Build history of the part. All positions in model axes, mm. A direction names the side the tool comes from. Coordinates: 2 decimals unless noted, no trailing zeros. Loops run counter-clockwise (first coordinate to the right, second up) from the corner with the lowest first, then second, coordinate; pieces in that order, holes last. Notation, with made-up numbers: (74.5, -32.75) -> (133.5, -32.75) arc R24 ccw to (133.5, -5.75) -> close; hole circle Ø3 at (29, 46.25). An arc over 180 degrees is marked (long way). One line per item, written item: value. Start each with the question number.
```python
from build123d import *

# Parameters (mm, degrees)
ESQUISSE6_R        = 25
ESQUISSE6_R_2      = 24
ESQUISSE8_R        = 26.000000000000004
ESQUISSE8_R_2      = 24.000000000000004
EXTRU_MINCE1_DEPTH = 1
EXTRU_MINCE2_START = 30
ESQUISSE9_R        = 26
ESQUISSE9_R_2      = 25
EXTRU_MINCE2_DEPTH = 30
CONG_1_R           = 1
CONG_2_R           = 1


with BuildPart() as part:
    # Balayage-Mince2: sweep along a path in Esquisse7
    with BuildLine(Plane(origin=(0, 0, 0), x_dir=(0, 0, -1), z_dir=(1, 0, 0))) as balayage_mince2_path:
        Line((0, 0), (-64.71019057874605, -6.94e-15))
        ThreePointArc((-64.71019057874605, -6.94e-15), (-69.91963590875396, 0.45576740963375073), (-74.97079487851613, 1.8092213764227365))
        Line((-74.97079487851613, 1.8092213764227365), (-106.64801221065042, 13.338785589701102))
    # Esquisse6 → Balayage-Mince2 (sweep)
    with BuildSketch(Plane.XY):
        Circle(ESQUISSE6_R)
        Circle(ESQUISSE6_R_2, mode=Mode.SUBTRACT)
    sweep(path=balayage_mince2_path.line)



with BuildPart() as body_2:
    # Esquisse8 → Extru.-Mince1 (new body)
    with BuildSketch(Plane(origin=(0, 35.836351928730004, 98.45956771981464), x_dir=(1, 0, 0), z_dir=(0, 0.34202014332566966, 0.9396926207859081))):
        with Locations((0, -23.94141003279684)):
            Circle(ESQUISSE8_R)
        with Locations((0, -23.94141003279684)):
            Circle(ESQUISSE8_R_2, mode=Mode.SUBTRACT)
    extrude(amount=EXTRU_MINCE1_DEPTH)


with BuildPart() as part_1:
    add(part.part)

    add(body_2.part)  # Extru.-Mince2 merges body 2
    # Esquisse9 → Extru.-Mince2 (add)
    with BuildSketch(Plane(origin=(0, 36.17837207205572, 99.39926034060053), x_dir=(1, 0, 0), z_dir=(0, 0.3420201433256696, 0.9396926207859081)).offset(EXTRU_MINCE2_START)):
        with Locations((0, -23.941410032796895)):
            Circle(ESQUISSE9_R)
        with Locations((0, -23.941410032796895)):
            Circle(ESQUISSE9_R_2, mode=Mode.SUBTRACT)
    extrude(amount=-EXTRU_MINCE2_DEPTH)

    # Congé1
    cong_1_edges = [part_1.edges().sort_by_distance(p)[0] for p in [
        (-25, 13.338785589701132, 106.6480122106504),
    ]]
    fillet(cong_1_edges, radius=CONG_1_R - 0.0001)  # a hair under: the kernel refuses the full size

    # Congé2
    cong_2_edges = [part_1.edges().sort_by_distance(p)[0] for p in [
        (-26.000000000000004, 13.33878558970111, 106.64801221065045),
    ]]
    fillet(cong_2_edges, radius=CONG_2_R)


solid = part_1.part
```
Item 1: Band-saw the part on A-A, the plane z = 50. List the corners of the cut face in (x, y), and give its area (3 significant figures).
Item 2: Tool access for faces 4 (the face through (-23.977, 1.055, 32.808)), 5 (the face through (-22.34, 22.49, 104.38)), 6 (the face through (-13.603, 43.963, 128.491)): list every direction of +Z, -Z, +X, -X, +Y, -Y with a clear straight run to the whole face (end or side of a thin tool).
Item 3: Probe probe 1 along Y at (x, z) = (0, 35); probe 2 along Y at (x, z) = (-4.5, 97); probe 3 along X at (y, z) = (3, 72). List the from-to ranges inside material, lowest first.
Item 4: Two-plate mould, pull along X, no slides. Class faces 1 (the face through (23.846, 25.939, 119.312)), 2 (the face through (-9.4, 22.3, 0)), 3 (the face through (12, -3, 129.2)): +X half, -X half, draft (parallel to the pull), parting line (faces both ways), or undercut.
Item 5: Drop flat-ended pins along their axis: pin 1 Ø3 at (x, z) = (13, 110) entering from +Y; pin 2 Ø4 at (x, z) = (-6.5, 83) entering from +Y; pin 3 Ø4 at (y, z) = (-16, 18) entering from +X. Give the stop position or say it passes through.
Worked out:
1. outline: circle Ø50 at (0, 0); hole circle Ø48 at (0, 0)
1. area: 154 mm²
2. face 4: -Z
2. face 5: none
2. face 6: +Z, +X, -X, +Y
3. probe 1: y = -25 to -24, 24 to 25
3. probe 2: y = -16.34 to -15.26, 34.91 to 36
3. probe 3: x = -24.92 to -23.91, 23.91 to 24.92
4. face 1: undercut
4. face 2: draft
4. face 3: parting line
5. pin 1: stops at y = 39.54
5. pin 2: stops at y = 31.32
5. pin 3: stops at x = 20.71
